Could you check a few things on this model? Use its own coordinates, in mm. A direction names the side the tool comes from. Round coordinates to 2 decimals unless told otherwise and drop trailing zeros. Write each loop counter-clockwise with the first axis right and the second up, starting at its lowest first coordinate (ties: lowest second). Pieces come first, ordered by that corner, then holes. Notation, with made-up numbers: (59.25, 70.25) -> (73.25, 70.25) arc R28 ccw to (73.25, 91.25) -> close; hole circle Ø3 at (-17.75, 38). An arc over 180 degrees is marked (long way). Answer as CSV lines item,"result". Start each with the question number.
Q1. For faces 4 (the flat face through (211.3, 184, 3)), 5 (the flat face through (109.2, 171, 3)), 6 (the flat face through (257, 92.75, 3)), 7 (the flat face through (64, 6, 3)), which set-ups out of +Z, -Z, +X, -X, +Y, -Y let a thin tool reach every point of the face, with its end or its side?
Q2. Will this pin go through, and if not, where does the flat tip stop? pin 1 Ø1 at (x, z) = (204, 1.5) entering from -Y.
Q3. If we mould it in two halves opening along X, with no side actions, what happens to faces 1 (the flat face through (267, 121.1, 3)), 2 (the flat face through (18.717, 3, 3)), 3 (the flat face through (220, 173.7, 3))? For each: pulls with the +X half, pulls with the -X half, needs draft (parallel to the pull), parting line crosses it, or undercut.
Q4. Imagine slicing it at B-B on z = 2.9. Give the number of separate pieces and of enclosed holes in the cut face, and give its area (3 significant figures).
Q5. If I drill on line 1 (Y direction, x = 196.8, z = 2); line 2 (Y direction, x = 84, z = 4.65); line 3 (Y direction, x = 209, z = 1.95), over which ranges is the centre line in solid material (lowest first)? Write a range as [from, to].
Q6. Imagine slicing it at A-A on y = 113.5. Please give me the cut outline in (x, z), and give its area (3 significant figures).
from build123d import *

# Parameters (mm, degrees)
ESBO_O1_W                = 270
ESBO_O1_H                = 187
RESSALTO_EXTRUS_O1_DEPTH = 6
ESBO_O2_W                = 30.1
ESBO_O2_H                = 6
ESBO_O2_W_2              = 20.2
ESBO_O2_W_3              = 62.783302492
ESBO_O2_W_4              = 18.716697508
CORTE_EXTRUS_O1_DEPTH    = 6
ESBO_O3_W                = 6
ESBO_O3_H                = 30.1
ESBO_O3_H_2              = 55.2
CORTE_EXTRUS_O2_DEPTH    = 6
ESBO_O4_W                = 0.75
ESBO_O4_H                = 15
ESBO_O4_W_2              = 1.5
ESBO_O4_W_3              = 15
ESBO_O4_H_2              = 1.5
CORTE_EXTRUS_O3_DEPTH    = 6
ESBO_O7_W                = 4.32
ESBO_O7_H                = 6
CORTE_EXTRUS_O4_DEPTH    = 194.4
ESBO_O8_W                = 30.4
ESBO_O8_H                = 6.4
ESBO_O8_R                = 1.75
CORTE_EXTRUS_O5_DEPTH    = 25.5
ESBO_O10_R               = 26.5
CORTE_EXTRUS_O6_DEPTH    = 25.5
FILETE1_R                = 0.75


with BuildPart() as part:
    # Esboço1 → Ressalto-extrusão1 (new body)
    with BuildSketch(Plane.XY):
        with Locations((135, 93.5)):
            Rectangle(ESBO_O1_W, ESBO_O1_H)
    extrude(amount=RESSALTO_EXTRUS_O1_DEPTH)

    # Esboço2 → Corte-extrusão1 (cut)
    with BuildSketch(Plane(origin=(0, 0, 0), x_dir=(-1, 0, 0), z_dir=(0, 0, -1))):
        with Locations((-256.15, 184)):
            Rectangle(ESBO_O2_W, ESBO_O2_H)
        with Locations((-201.2, 184)):
            Rectangle(ESBO_O2_W_2, ESBO_O2_H)
        with Locations((-129.908348754, 184)):
            Rectangle(ESBO_O2_W_3, ESBO_O2_H)
        with Locations((-58.616697508, 184)):
            Rectangle(ESBO_O2_W_2, ESBO_O2_H)
        with Locations((-9.358348754, 184)):
            Rectangle(ESBO_O2_W_4, ESBO_O2_H)
        with Locations((-9.358348754, 3)):
            Rectangle(ESBO_O2_W_4, ESBO_O2_H)
        with Locations((-58.616697508, 3)):
            Rectangle(ESBO_O2_W_2, ESBO_O2_H)
        with Locations((-129.908348754, 3)):
            Rectangle(ESBO_O2_W_3, ESBO_O2_H)
        with Locations((-201.2, 3)):
            Rectangle(ESBO_O2_W_2, ESBO_O2_H)
        with Locations((-256.15, 3)):
            Rectangle(ESBO_O2_W, ESBO_O2_H)
    extrude(amount=-CORTE_EXTRUS_O1_DEPTH, mode=Mode.SUBTRACT)

    # Esboço3 → Corte-extrusão2 (cut)
    with BuildSketch(Plane.XY.offset(6)):
        with Locations((267, 165.95)):
            Rectangle(ESBO_O3_W, ESBO_O3_H)
        with Locations((267, 93.5)):
            Rectangle(ESBO_O3_W, ESBO_O3_H_2)
        with Locations((267, 21.05)):
            Rectangle(ESBO_O3_W, ESBO_O3_H)
    extrude(amount=-CORTE_EXTRUS_O2_DEPTH, mode=Mode.SUBTRACT)

    # Esboço4 → Corte-extrusão3 (cut)
    with BuildSketch(Plane.XY.offset(6)):
        with Locations((58.241697508, 173.5)):
            Rectangle(ESBO_O4_W, ESBO_O4_H)
        with Locations((58.991697508, 173.5)):
            Rectangle(ESBO_O4_W, ESBO_O4_H)
        with Locations((58.241697508, 13.5)):
            Rectangle(ESBO_O4_W, ESBO_O4_H)
        with Locations((58.991697508, 13.5)):
            Rectangle(ESBO_O4_W, ESBO_O4_H)
        with Locations((201.2, 13.5)):
            Rectangle(ESBO_O4_W_2, ESBO_O4_H)
        with Locations((256.5, 93.5)):
            Rectangle(ESBO_O4_W_3, ESBO_O4_H_2)
        with Locations((201.2, 173.5)):
            Rectangle(ESBO_O4_W_2, ESBO_O4_H)
    extrude(amount=-CORTE_EXTRUS_O3_DEPTH, mode=Mode.SUBTRACT)

    # Esboço7 → Corte-extrusão4 (cut)
    with BuildSketch(Plane(origin=(0, 6, 0), x_dir=(1, 0, 0), z_dir=(0, 1, 0))):
        with Locations((2.16, -3)):
            Rectangle(ESBO_O7_W, ESBO_O7_H)
    extrude(amount=CORTE_EXTRUS_O4_DEPTH, mode=Mode.SUBTRACT)

    # Esboço8 → Corte-extrusão5 (cut)
    with BuildSketch(Plane.XY.offset(6)):
        with Locations((94, 30.5)):
            Rectangle(ESBO_O8_W, ESBO_O8_H)
        with Locations((94, 16.5)):
            Rectangle(ESBO_O8_W, ESBO_O8_H)
        with Locations((220, 16.5)):
            Rectangle(ESBO_O8_W, ESBO_O8_H)
        with Locations((220, 30.5)):
            Rectangle(ESBO_O8_W, ESBO_O8_H)
        with Locations((117.2, 30.5)):
            Circle(ESBO_O8_R)
        with Locations((117.2, 16.5)):
            Circle(ESBO_O8_R)
        with Locations((196.8, 30.5)):
            Circle(ESBO_O8_R)
        with Locations((196.8, 16.5)):
            Circle(ESBO_O8_R)
    corte_extrus_o5 = extrude(amount=-CORTE_EXTRUS_O5_DEPTH, mode=Mode.SUBTRACT)

    # Espelhar1: Corte-extrusão5 across plane
    add(corte_extrus_o5.mirror(Plane(origin=(0, 93.5, 0), x_dir=(0, 0, 1), z_dir=(0, -1, 0))), mode=Mode.SUBTRACT)

    # Esboço10 → Corte-extrusão6 (cut)
    with BuildSketch(Plane.XY.offset(6)):
        with Locations((84, 93.5)):
            Circle(ESBO_O10_R)
    extrude(amount=-CORTE_EXTRUS_O6_DEPTH, mode=Mode.SUBTRACT)

    # Filete1
    filete1_edges = [part.edges().sort_by_distance(p)[0] for p in [
        (59.366697508, 166, 3),
        (57.866697508, 166, 3),
        (200.45, 166, 3),
        (201.95, 166, 3),
        (249, 92.75, 3),
        (249, 94.25, 3),
        (201.95, 21, 3),
        (200.45, 21, 3),
        (57.866697508, 21, 3),
        (59.366697508, 21, 3),
    ]]
    fillet(filete1_edges, radius=FILETE1_R - 0.0001)  # a hair under: the kernel refuses the full size


solid = part.part
Checks:
1,face 4,"+Z, -Z, +Y"
1,face 5,"+Z, -Z"
1,face 6,"+Z, -Z, +X"
1,face 7,"+Z, -Z, -Y"
2,pin 1,"y = 6"
3,face 1,"needs draft"
3,face 2,"pulls with the -X half"
3,face 3,"undercut"
4,separate pieces,"1"
4,enclosed holes,"17"
4,area,"43,300 mm^2"
5,line 1,"[6, 14.75], [18.25, 28.75], [32.25, 154.75], [158.25, 168.75], [172.25, 181]"
5,line 2,"[0, 13.3], [19.7, 27.3], [33.7, 67], [120, 153.3], [159.7, 167.3], [173.7, 187]"
5,line 3,"[6, 13.3], [19.7, 27.3], [33.7, 153.3], [159.7, 167.3], [173.7, 181]"
6,outline,"(4.32, 0) -> (66.61, 0) -> (66.61, 6) -> (4.32, 6) -> close; (101.39, 0) -> (264, 0) -> (264, 6) -> (101.39, 6) -> close"
6,area,"1,350 mm^2"
